Study the drawing (mm; zero at the part's minimum x, y, z) and answer. Coordinates: 2 decimals unless noted, no trailing zeros. Loops run counter-clockwise (first coordinate to the right, second up) from the corner with the lowest first, then second, coordinate; pieces in that order, holes last. Notation, with made-up numbers: (34.5, -34.75) -> (76.5, -34.75) arc R14 ccw to (76.5, -27.75) -> close; hole circle Ø8 at (-10.75, 57). An arc over 180 degrees is marked (long way). One line per question, with ' | ' between items.
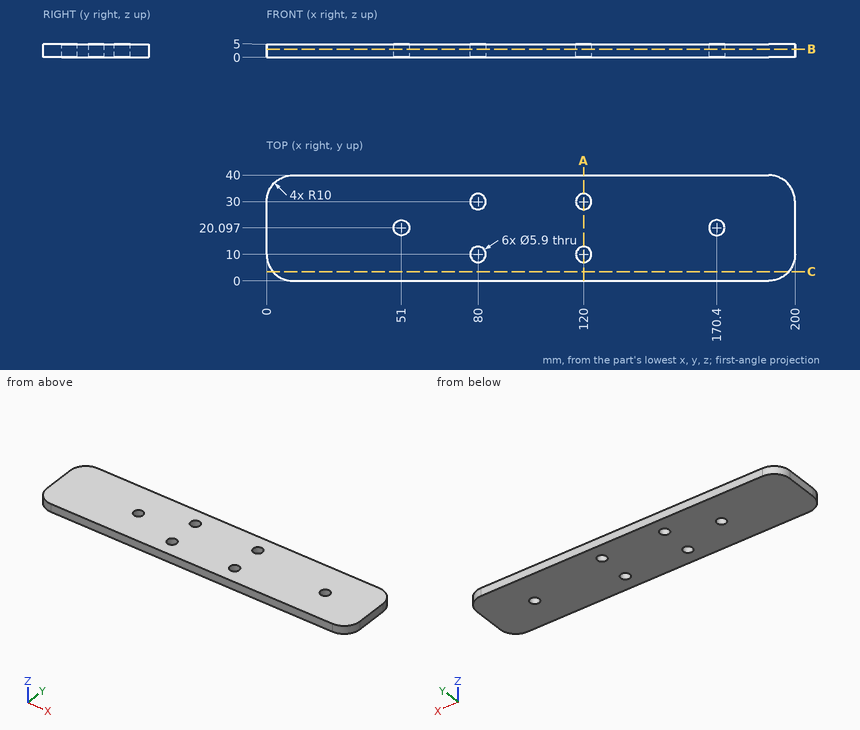
1) Find section B-B (z = 3.05). Write down the section's boundary in (x, y), plus the area to 3 significant figures.
Check values:
outline: (0, 10) arc R10 ccw to (10, 0) -> (190, 0) arc R10 ccw to (200, 10) -> (200, 30) arc R10 ccw to (190, 40) -> (10, 40) arc R10 ccw to (0, 30) -> close; hole circle Ø5.9 at (51, 20.1); hole circle Ø5.9 at (80, 10); hole circle Ø5.9 at (80, 30); hole circle Ø5.9 at (120, 10); hole circle Ø5.9 at (120, 30); hole circle Ø5.9 at (170.4, 20.1) | area: 7,750 mm^2
2) Flat-ended cylindrical pins translate along their axes: pin 1 (7.5 mm diameter, centred on x = 120, y = 10, fed in from +Z); pin 2 (3.5 mm diameter, centred on x = 80, y = 10, fed in from +Z). Find the tip coordinate at first contact, or state that the pin passes through.
Check values:
pin 1: stops at z = 5 | pin 2: passes through
3) Find section C-C (y = 3.5). Write down the section's boundary in (x, z).
Check values:
outline: (2.4, 0) -> (197.6, 0) -> (197.6, 5) -> (2.4, 5) -> close
4) Find the intervals of material crossed by line 1 along Y through (x, z) = (80, 2.9); line 2 along X through (y, z) = (18.5, 0.6); line 3 along X through (y, z) = (10.5, 0.6), in increasing order.
Check values:
line 1: y = 0 to 7.05, 12.95 to 27.05, 32.95 to 40 | line 2: x = 0 to 48.52, 53.48 to 167.92, 172.88 to 200 | line 3: x = 0 to 77.09, 82.91 to 117.09, 122.91 to 200
5) Find section A-A (x = 120). Write down the section's boundary in (y, z).
Check values:
outline: (0, 0) -> (7.05, 0) -> (7.05, 5) -> (0, 5) -> close; (12.95, 0) -> (27.05, 0) -> (27.05, 5) -> (12.95, 5) -> close; (32.95, 0) -> (40, 0) -> (40, 5) -> (32.95, 5) -> close
